Study the drawing (mm; zero at the part's minimum x, y, z) and answer. A direction names the side the tool comes from. Round coordinates to 2 decimals unless told otherwise and drop trailing zeros. Loops run counter-clockwise (first coordinate to the right, second up) from the corner with the lowest first, then second, coordinate; pieces in that order, holes last. Notation, with made-up numbers: (13, 33.25) - (27, 33.25) arc R23 ccw to (27, 72.25) - close; hole circle Ø4 at (38, 2.5). An arc over 180 degrees is marked (long way). One line per item, written item: value.
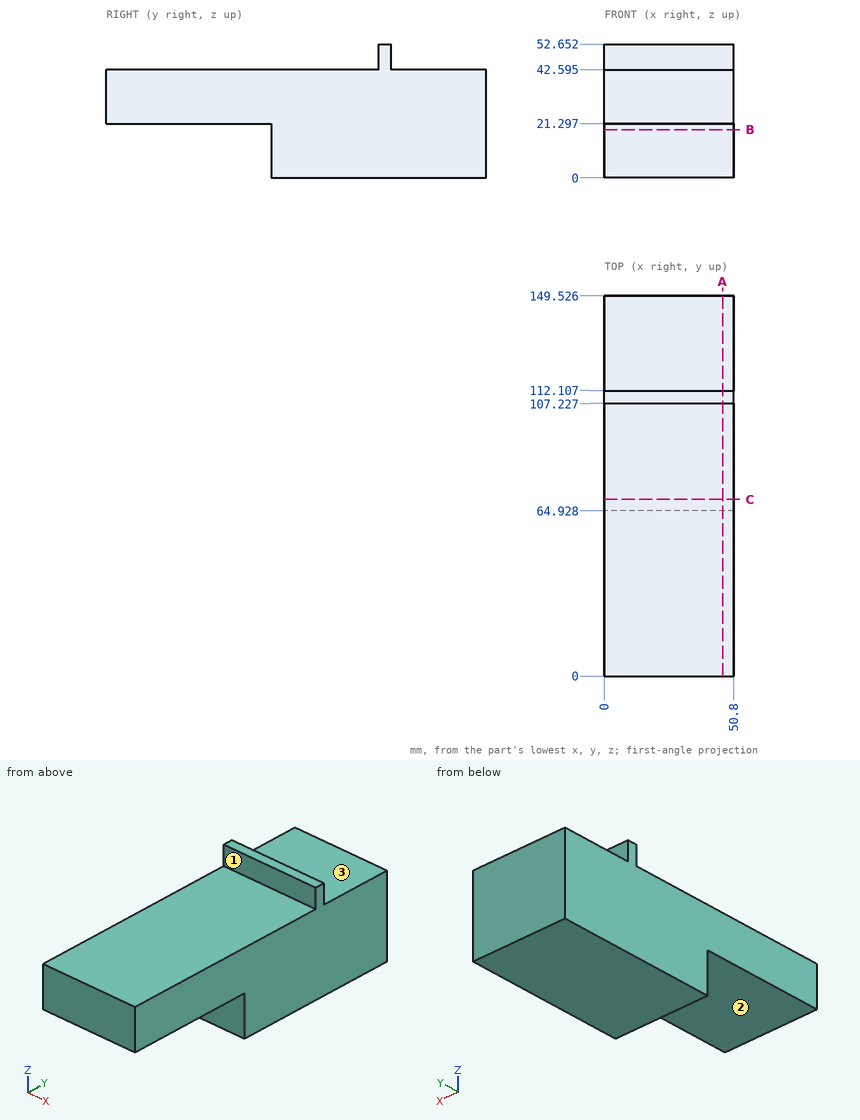
1) A cutting plane is placed at A-A on x = 46.5. Give the vertices of the cut face in (y, z) (1 decimal).
Final values:
outline: (0, 21.3) - (64.9, 21.3) - (64.9, 0) - (149.5, 0) - (149.5, 42.6) - (112.1, 42.6) - (112.1, 52.7) - (107.2, 52.7) - (107.2, 42.6) - (0, 42.6) - close
2) A cutting plane is placed at B-B on z = 19. Give the vertices of the cut face in (x, y) (1 decimal), and give its area (3 significant figures).
Final values:
outline: (0, 64.9) - (50.8, 64.9) - (50.8, 149.5) - (0, 149.5) - close
area: 4,300 mm2
3) Each of these flat-tipped pins is pushed along its axis until it touches: pin 1 Ø1.5 at (y, z) = (129, 20) entering from -X; pin 2 Ø2 at (x, y) = (45.5, 35.5) entering from -Z; pin 3 Ø5 at (x, y) = (19.5, 120) entering from +Z (1 decimal); pin 4 Ø4 at (x, z) = (38, 19) entering from -Y. Where does it stop, or does it pass through?
Final values:
pin 1: x = 0
pin 2: z = 21.3
pin 3: z = 42.6
pin 4: y = 64.93
4) For the marked faces 1, 2 and 3, determine the directions among +Z, -Z, +X, -X, +Y, -Y from which every point of the face is accessible in a straight line to the end or side of a thin tool.
Final values:
face 1: +Z, +X, -X, -Y
face 2: -Z, +X, -X, -Y
face 3: +Z, +X, -X, +Y
5) Consider L1, parallel to Z at x = 15, y = 28 (1 decimal); L2, parallel to Y at x = 21, z = 8 (1 decimal); L3, parallel to Z at x = 36.5, y = 134.5 (1 decimal). Determine where each line is inside the solid, lowest interval first.
Final values:
L1: 21.3 to 42.6
L2: 64.9 to 149.5
L3: 0 to 42.6
6) A cutting plane is placed at C-C on y = 69.5. Give the vertices of the cut face in (x, z) (1 decimal), and give its area (3 significant figures).
Final values:
outline: (0, 0) - (50.8, 0) - (50.8, 42.6) - (0, 42.6) - close
area: 2,160 mm2
